```python
from build123d import *

# Parameters (mm, degrees)
SKETCH3_W = 1.3
SKETCH3_H = 0.473161305


with BuildPart() as part:
    # Sketch2 → Body (revolve)
    with BuildSketch(Plane(origin=(0, 0, 0), x_dir=(0, 0, -1), z_dir=(1, 0, 0))):
        with BuildLine():
            Line((-15.645349183, 10.053677391), (-16, 10.053677391))
            Line((-16, 10.053677391), (-16, 10.526838695))
            ThreePointArc((-16, 10.526838695), (-15.861414262, 10.861414262), (-15.526838695, 11))
            Line((-15.526838695, 11), (15.526838695, 11))
            ThreePointArc((15.526838695, 11), (15.861414262, 10.861414262), (16, 10.526838695))
            Line((16, 10.526838695), (16, 10.053677391))
            Line((16, 10.053677391), (15.645349183, 10.053677391))
            Line((15.645349183, 10.053677391), (15.645349183, 6))
            Line((15.645349183, 6), (-15.645349183, 6))
            Line((-15.645349183, 6), (-15.645349183, 10.053677391))
        make_face()
    revolve(axis=Axis((0, 0, 16), (0, 0, -1)))

    # Sketch3 → Track (revolve, cut)
    with BuildSketch(Plane(origin=(0, 0, 0), x_dir=(0, 0, -1), z_dir=(1, 0, 0))):
        with Locations((10.8, 10.763419348)):
            Rectangle(SKETCH3_W, SKETCH3_H)
        with Locations((-10.8, 10.763419348)):
            Rectangle(SKETCH3_W, SKETCH3_H)
    revolve(axis=Axis((0, 0, 16), (0, 0, -1)), mode=Mode.SUBTRACT)


solid = part.part
```
Verification items for the finished model (mm, model axes). A direction names the side the tool comes from. Round coordinates to 2 decimals unless told otherwise and drop trailing zeros. Write each loop counter-clockwise with the first axis right and the second up, starting at its lowest first coordinate (ties: lowest second). Pieces come first, ordered by that corner, then holes. Notation, with made-up numbers: (18.5, 36.5) - (46.5, 36.5) arc R19 cw to (46.5, 66.5) - close; hole circle Ø10 at (-33.75, 68.5). An arc over 180 degrees is marked (long way). Answer as a JSON object with one key per item and string values. Group by question number.
Q1. Tool access check on faces 4 (the cylindrical face through (-10.277, -2.282, -10.809)), 5 (the flat face through (-7, 0, 15.645)), 6 (the cylindrical face through (0, -6, 0)), 7 (the cylindrical face through (-9.815, -2.179, -15.82)). Record the directions out of +Z, -Z, +X, -X, +Y, -Y that give a thin tool (end or side, any length) a straight path to the whole face; none if there is none.
Q2. Go/stop test with flat-tipped pins: pin 1 Ø2 at (x, y) = (-7.5, 2.5) entering from +Z; pin 2 Ø10 at (x, y) = (-2, 3.5) entering from -Z; pin 3 Ø4 at (y, z) = (-4.5, 4) entering from +X. Record where each tip stops, or that it passes through.
Q3. Mould release check, pull along X, two halves, no side actions. Record for faces 1 (the cylindrical face through (-10.74, -2.38, -0.14)), 2 (the flat face through (-7, 0, -15.645)), 3 (the flat face through (-6, -9, -10.15)): released by +X, released by -X, zero draft, split by the parting line, or undercut.
Q4. Thickness scan on line 1 (X direction, y = 0, z = 4.5); line 2 (X direction, y = -2.5, z = 4); line 3 (Z direction, x = 0.25, y = -9). Record the ranges inside material, lowest first.
Q5. Section check A-A, the plane z = -14. Enter the section's corners in (x, y).
Found:
{
 "1": {"face 4": "none", "face 5": "+Z", "face 6": "+Z, -Z", "face 7": "-Z"},
 "2": {"pin 1": "stops at z = 15.65", "pin 2": "stops at z = -15.65", "pin 3": "stops at x = 10.71"},
 "3": {"face 1": "split by the parting line", "face 2": "undercut", "face 3": "zero draft"},
 "4": {"line 1": "x = -11 to -6, 6 to 11", "line 2": "x = -10.71 to -5.45, 5.45 to 10.71", "line 3": "z = -15.65 to 15.65"},
 "5": {"outline": "circle Ø22 at (0, 0); hole circle Ø12 at (0, 0)"}
}
